Part model, mm, in its own coordinate system. Round coordinates to 2 decimals unless told otherwise and drop trailing zeros. Write each loop counter-clockwise with the first axis right and the second up, starting at its lowest first coordinate (ties: lowest second). Pieces come first, ordered by that corner, then holes. Notation, with made-up numbers: M 10,36 L 52,36 A29 cw 52,60 Z; hole C 56,59 d8. An arc over 180 degrees is marked long. Use a Markdown table: item, result. Add a question column.
1) Slice it at A-A on y = 12.62. Write the cut outline in (x, z).
2) Wall check: probe 1 along Y at (x, z) = (12.7, 1.1); probe 2 along X at (y, z) = (28, 1.1); probe 3 along Y at (x, z) = (17, 1). Give the ranges that are in metal, low to high.
3) Slice it at B-B on y = 2.54. Write the cut outline in (x, z), plus the area to 3 significant figures.
4) Slice it at C-C on z = 0.3. Give the number of separate pieces and of enclosed holes in the cut face, plus the area to 3 significant figures.
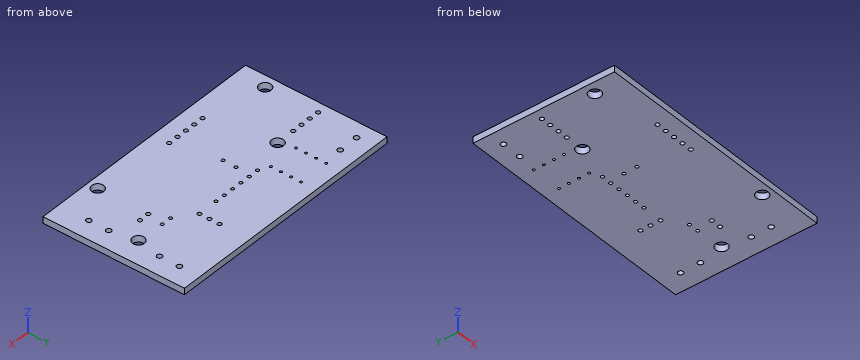
Autodesk Inventor part; units mm, degrees
ref_plane "YZ Plane" through (0, 0, 0) normal (1, 0, 0) x (0, 1, 0)
ref_plane "XZ Plane" through (0, 0, 0) normal (0, 1, 0) x (-1, 0, 0)
ref_plane "XY Plane" through (0, 0, 0) normal (0, 0, 1) x (1, 0, 0)
sketch "Эскиз1" plane through (0, 0, 0) normal (0, 0, 1) x (1, 0, 0)
  line L0 (-8.89, 0) -> (53.01, 0)
  line L1 (53.01, 0) -> (53.01, 35.55)
  line L2 (53.01, 35.55) -> (-8.89, 35.55)
  line L3 (-8.89, 35.55) -> (-8.89, 0)
  circle A0 centre (15.24, 22.86) radius 0.405
  circle A1 centre (17.78, 22.86) radius 0.405
  circle A2 centre (20.32, 22.86) radius 0.405
  circle A3 centre (22.86, 22.86) radius 0.405
  circle A4 centre (25.4, 22.86) radius 0.405
  circle A5 centre (27.94, 22.86) radius 0.405
  circle A6 centre (37.62, 19.41) radius 0.405
  circle A7 centre (40.16, 19.41) radius 0.405
  circle A8 centre (0.1, 31.17) radius 0.65
  circle A9 centre (-4.9, 31.17) radius 0.65
  circle A10 centre (1.27, 20.32) radius 0.51
  circle A11 centre (-1.27, 20.32) radius 0.51
  circle A12 centre (-3.81, 20.32) radius 0.51
  circle A13 centre (-6.35, 20.32) radius 0.51
  circle A14 centre (48.26, 25.4) radius 0.65
  circle A15 centre (48.26, 30.4) radius 0.65
  circle A16 centre (9.33, 4.16) radius 0.51
  circle A17 centre (11.87, 4.16) radius 0.51
  circle A18 centre (14.41, 4.16) radius 0.51
  circle A19 centre (16.95, 4.16) radius 0.51
  circle A20 centre (19.49, 4.16) radius 0.51
  circle A21 centre (39.37, 15.24) radius 0.51
  circle A22 centre (41.91, 15.24) radius 0.51
  circle A23 centre (48.26, 7.62) radius 0.65
  circle A24 centre (48.26, 12.62) radius 0.65
  circle A25 centre (12.7, 24.13) radius 0.3
  circle A26 centre (5.08, 26.67) radius 0.3
  circle A27 centre (5.08, 24.13) radius 0.3
  circle A28 centre (12.7, 26.67) radius 0.3
  circle A29 centre (5.08, 31.75) radius 0.3
  circle A30 centre (5.08, 29.21) radius 0.3
  circle A31 centre (12.7, 29.21) radius 0.3
  circle A32 centre (12.7, 31.75) radius 0.3
  circle A33 centre (33.02, 25.4) radius 0.5
  circle A34 centre (33.02, 27.94) radius 0.5
  circle A35 centre (33.02, 22.86) radius 0.5
  circle A36 centre (-5.9225, 7.3465) radius 1.5
  circle A37 centre (39.37, 2.54) radius 1.5
  circle A38 centre (46.99, 19.05) radius 1.5
  circle A39 centre (6.0563, 20.3433) radius 1.5
  circle A40 centre (17.1236, 18.9948) radius 0.4
  circle A41 centre (17.0778, 15.6995) radius 0.4
extrude "OmniBot_motor_driver.brdКонтур" add sketch "Эскиз1" along normal blind 1.6
properties part number "OmniBot_motor_driver.brdКонтур"
Entries:
| question | item | result |
|---|---|---|
| 1 | outline | M -8.89,0 L 47.61,0 L 47.61,1.6 L -8.89,1.6 Z; M 48.91,0 L 53.01,0 L 53.01,1.6 L 48.91,1.6 Z |
| 2 | probe 1 | y = 0 to 23.83, 24.43 to 26.37, 26.97 to 28.91, 29.51 to 31.45, 32.05 to 35.55 |
| 2 | probe 2 | x = -8.89 to 32.52, 33.52 to 53.01 |
| 2 | probe 3 | y = 0 to 3.65, 4.67 to 15.31, 16.09 to 18.61, 19.38 to 35.55 |
| 3 | outline | M -8.89,0 L 37.87,0 L 37.87,1.6 L -8.89,1.6 Z; M 40.87,0 L 53.01,0 L 53.01,1.6 L 40.87,1.6 Z |
| 3 | area | 94.2 mm^2 |
| 4 | separate pieces | 1 |
| 4 | enclosed holes | 42 |
| 4 | area | 2,150 mm^2 |
